Source: CAD feature listing. Evaluate the final solid. Frame: model axes, mm. Face numbers are marked on the shaded views. A direction names the side the tool comes from. Give positions to 0.01 mm unless a question says otherwise; leave off trailing zeros. Order: outer loops, then holes, each group sorted by start corner. A loop starts at its lowest first (then second) coordinate and runs counter-clockwise, first axis right, second up. Notation, with made-up numbers: (78, 11) - (107, 11) arc R21 cw to (107, 43) - close; hole circle Ø1 at (-26.5, 59.5). An arc over 180 degrees is marked (long way). Use CSV: the item, a comma, the result in double quotes.
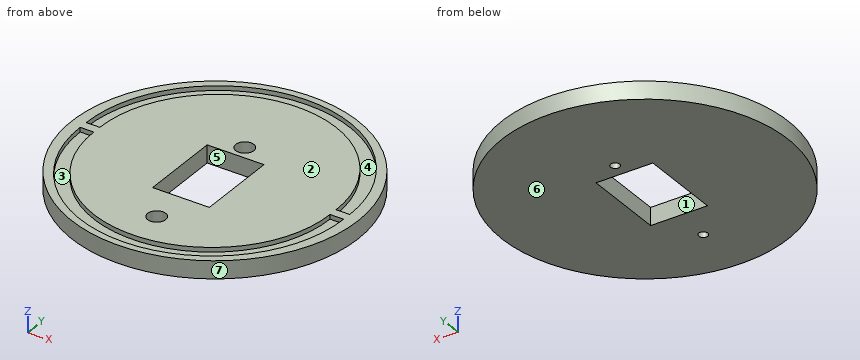
```python
from build123d import *

# Parameters (mm, degrees)
CROQUIS1_R              = 31.5
SALIENTE_EXTRUIR1_DEPTH = 2.4
CROQUIS2_W              = 16.1
CROQUIS2_H              = 36.6
CROQUIS2_W_2            = 12.5
CROQUIS2_H_2            = 33
SALIENTE_EXTRUIR2_DEPTH = 22.5
CROQUIS5_W              = 16.1
CROQUIS5_H              = 36.6
CORTAR_EXTRUIR2_DEPTH   = 9
CROQUIS6_R              = 1.5
CORTAR_EXTRUIR3_DEPTH   = 2.4
CROQUIS7_W              = 12.5
CROQUIS7_H              = 9
SALIENTE_EXTRUIR3_DEPTH = 33
CROQUIS8_R              = 1
CORTAR_EXTRUIR5_DEPTH   = 9
SALIENTE_EXTRUIR4_DEPTH = 12.5
CROQUIS10_W             = 4
CROQUIS10_H             = 2
CORTAR_EXTRUIR6_DEPTH   = 9
CROQUIS11_R             = 31.5
CROQUIS11_W             = 12.5
CROQUIS11_H             = 18
SALIENTE_EXTRUIR5_DEPTH = 3.9
CORTAR_EXTRUIR7_START   = 7
CROQUIS12_R             = 1
CORTAR_EXTRUIR7_DEPTH   = 3.9
CROQUIS13_R             = 2
CORTAR_EXTRUIR8_DEPTH   = 2.4
CROQUIS14_R             = 31.5
CORTAR_EXTRUIR9_DEPTH   = 24.9
CROQUIS15_R             = 31.5
CROQUIS15_R_2           = 2
CROQUIS15_W             = 12.5
CROQUIS15_H             = 18
SALIENTE_EXTRUIR6_DEPTH = 1
CORTAR_EXTRUIR10_DEPTH  = 2
CROQUIS17_R             = 31.5
CORTAR_EXTRUIR11_DEPTH  = 1


with BuildPart() as part:
    # Croquis1 → Saliente-Extruir1 (new body)
    with BuildSketch(Plane.XY):
        with Locations((-51.235671923, 9.786589019)):
            Circle(CROQUIS1_R)
    extrude(amount=SALIENTE_EXTRUIR1_DEPTH)

    # Croquis2 → Saliente-Extruir2 (add)
    with BuildSketch(Plane.XY.offset(2.4)):
        with Locations((-51.235671923, 5.086589019)):
            Rectangle(CROQUIS2_W, CROQUIS2_H)
        with Locations((-51.235671923, 5.086589019)):
            Rectangle(CROQUIS2_W_2, CROQUIS2_H_2, mode=Mode.SUBTRACT)
    extrude(amount=SALIENTE_EXTRUIR2_DEPTH)

    # Croquis5 → Cortar-Extruir2 (cut)
    with BuildSketch(Plane.XY.offset(2.4)):
        with Locations((-51.235671923, 5.086589019)):
            Rectangle(CROQUIS5_W, CROQUIS5_H)
    extrude(amount=-CORTAR_EXTRUIR2_DEPTH, mode=Mode.SUBTRACT)


with BuildPart() as cortar_extruir2_piece_1:
    # of the separate pieces the step leaves, piece 1, a body of its own (cortar_extruir2_pieces)
    add(part.part.solids().sort_by_distance((-19.735671923, 9.786589019, 0))[0])

    # Croquis6 → Cortar-Extruir3 (cut)
    with BuildSketch(Plane(origin=(0, 0, 0), x_dir=(-1, 0, 0), z_dir=(0, 0, -1))):
        with Locations((34.618662565, 26.403598377)):
            Circle(CROQUIS6_R)
        with Locations((67.85268128, 26.403598377)):
            Circle(CROQUIS6_R)
        with Locations((67.85268128, -6.830420339)):
            Circle(CROQUIS6_R)
        with Locations((34.618662565, -6.830420339)):
            Circle(CROQUIS6_R)
        Polygon((51.235671923, 23.386589019), (53.235671923, 23.386589019), (53.235671923, 43.386589019), (49.235671923, 43.386589019), (49.235671923, 23.386589019), align=None)
    extrude(amount=-CORTAR_EXTRUIR3_DEPTH, mode=Mode.SUBTRACT)


with BuildPart() as cortar_extruir2_piece_2:
    # of the separate pieces the step leaves, piece 2, a body of its own (cortar_extruir2_pieces)
    add(part.part.solids().sort_by_distance((-59.285671923, -13.213410981, 24.9))[0])

    # Croquis7 → Saliente-Extruir3 (add)
    with BuildSketch(Plane.XZ.offset(-21.586589019)):
        with Locations((-51.235671923, 13.4)):
            Rectangle(CROQUIS7_W, CROQUIS7_H)
    extrude(amount=SALIENTE_EXTRUIR3_DEPTH)

    # Croquis8 → Cortar-Extruir5 (cut)
    with BuildSketch(Plane.XY.offset(17.9)):
        with Locations((-51.235671923, -9.413410981)):
            Circle(CROQUIS8_R)
        with Locations((-51.235671923, 19.636589019)):
            Circle(CROQUIS8_R)
        Polygon((-44.985671923, -6.413410981), (-57.485671923, -6.413410981), (-57.485671923, 16.586589019), (-53.235671923, 16.586589019), (-53.235671923, 18.586589019), (-49.235671923, 18.586589019), (-49.235671923, 16.586589019), (-44.985671923, 16.586589019), align=None)
    extrude(amount=-CORTAR_EXTRUIR5_DEPTH, mode=Mode.SUBTRACT)

    # Croquis9 → Saliente-Extruir4 (add)
    with BuildSketch(Plane.ZY.offset(44.985671923)):
        Polygon((8.9, -6.413410981), (3.9, -11.413410981), (8.9, -11.413410981), align=None)
        Polygon((8.9, 16.586589019), (3.9, 21.586589019), (8.9, 21.586589019), align=None)
    extrude(amount=SALIENTE_EXTRUIR4_DEPTH)

    # Croquis10 → Cortar-Extruir6 (cut)
    with BuildSketch(Plane.XY.offset(8.9)):
        with Locations((-51.235671923, 17.586589019)):
            Rectangle(CROQUIS10_W, CROQUIS10_H)
    extrude(amount=-CORTAR_EXTRUIR6_DEPTH, mode=Mode.SUBTRACT)

    # Croquis11 → Saliente-Extruir5 (add)
    with BuildSketch(Plane.XY.offset(24.9)):
        with Locations((-51.235671923, 9.786589019)):
            Circle(CROQUIS11_R)
        with Locations((-51.235671923, 7.586589019)):
            Rectangle(CROQUIS11_W, CROQUIS11_H, mode=Mode.SUBTRACT)
    extrude(amount=SALIENTE_EXTRUIR5_DEPTH)

    # Croquis12 → Cortar-Extruir7 (cut)
    with BuildSketch(Plane.XY.offset(17.9).offset(CORTAR_EXTRUIR7_START)):
        with Locations((-51.235671923, 19.636589019)):
            Circle(CROQUIS12_R)
        with Locations((-51.235671923, -9.413410981)):
            Circle(CROQUIS12_R)
    extrude(amount=CORTAR_EXTRUIR7_DEPTH, mode=Mode.SUBTRACT)

    # Croquis13 → Cortar-Extruir8 (cut)
    with BuildSketch(Plane.XY.offset(28.8)):
        with Locations((-51.235671923, 19.636589019)):
            Circle(CROQUIS13_R)
        with Locations((-51.235671923, -9.413410981)):
            Circle(CROQUIS13_R)
    extrude(amount=-CORTAR_EXTRUIR8_DEPTH, mode=Mode.SUBTRACT)


with BuildPart() as cortar_extruir9_tool:
    # Croquis14 → Cortar-Extruir9 (new body)
    with BuildSketch(Plane(origin=(0, 0, 0), x_dir=(-1, 0, 0), z_dir=(0, 0, -1))):
        with Locations(Location((51.235671923, 9.786589019, 0), (0, 0, 180))):
            Circle(CROQUIS14_R)
    extrude(amount=-CORTAR_EXTRUIR9_DEPTH)


with BuildPart() as cortar_extruir2_piece_1_1:
    add(cortar_extruir2_piece_1.part)

    # Cortar-Extruir9: cut by cortar_extruir9_tool
    add(cortar_extruir9_tool.part, mode=Mode.SUBTRACT)


with BuildPart() as cortar_extruir2_piece_2_1:
    add(cortar_extruir2_piece_2.part)

    # Cortar-Extruir9: cut by cortar_extruir9_tool
    add(cortar_extruir9_tool.part, mode=Mode.SUBTRACT)

    # Croquis15 → Saliente-Extruir6 (add)
    with BuildSketch(Plane.XY.offset(28.8)):
        with Locations((-51.235671923, 9.786589019)):
            Circle(CROQUIS15_R)
        with Locations((-51.235671923, 19.636589019)):
            Circle(CROQUIS15_R_2, mode=Mode.SUBTRACT)
        with Locations((-51.235671923, -9.413410981)):
            Circle(CROQUIS15_R_2, mode=Mode.SUBTRACT)
        with Locations((-51.235671923, 7.586589019)):
            Rectangle(CROQUIS15_W, CROQUIS15_H, mode=Mode.SUBTRACT)
    extrude(amount=SALIENTE_EXTRUIR6_DEPTH)

    # Croquis16 → Cortar-Extruir10 (cut)
    with BuildSketch(Plane.XY.offset(29.8)):
        with BuildLine():
            Line((-22.235671923, 8.786589019), (-25.235671923, 8.786589019))
            ThreePointArc((-25.235671923, 8.786589019), (-51.235671923, -17.213410981), (-77.235671923, 8.786589019))
            Line((-77.235671923, 8.786589019), (-80.235671923, 8.786589019))
            ThreePointArc((-80.235671923, 8.786589019), (-51.235671923, -20.213410981), (-22.235671923, 8.786589019))
        make_face()
        with BuildLine():
            Line((-22.235671923, 10.786589019), (-25.235671923, 10.786589019))
            ThreePointArc((-25.235671923, 10.786589019), (-51.235671923, 36.786589019), (-77.235671923, 10.786589019))
            Line((-77.235671923, 10.786589019), (-80.235671923, 10.786589019))
            ThreePointArc((-80.235671923, 10.786589019), (-51.235671923, 39.786589019), (-22.235671923, 10.786589019))
        make_face()
    extrude(amount=-CORTAR_EXTRUIR10_DEPTH, mode=Mode.SUBTRACT)

    # Croquis17 → Cortar-Extruir11 (cut)
    with BuildSketch(Plane.XY.offset(29.8)):
        with Locations((-51.235671923, 9.786589019)):
            Circle(CROQUIS17_R)
    extrude(amount=-CORTAR_EXTRUIR11_DEPTH, mode=Mode.SUBTRACT)


solid = cortar_extruir2_piece_2_1.part
```
Item 1: First-contact query: pin 1 (1.2 mm diameter, centred on x = -51, y = -8.5, fed in from +Z); pin 2 (0.5 mm diameter, centred on x = -78.5, z = 28.5, fed in from -Y). Flat tips, straight axial feed; report the tip coordinate or a pass-through.
Filled in:
pin 1,"stops at z = 26.4"
pin 2,"stops at y = -6.41"
Item 2: Set-up query: the marked faces 1, 2 and 3. Return all of +Z, -Z, +X, -X, +Y, -Y with unobstructed straight access to the full face (end or side cutting, diameter ignored); none if empty.
Filled in:
face 1,"+Z, -Z"
face 2,"+Z, +X, -X, +Y, -Y"
face 3,"+Z"
Item 3: Section D-D on x = -48. Return the cut outline in (y, z), then the cut area to 3 significant figures.
Filled in:
outline,"(-21.55, 24.9) - (-1.41, 24.9) - (-1.41, 28.8) - (-17.01, 28.8) - (-17.01, 27.8) - (-20.03, 27.8) - (-20.03, 28.8) - (-21.55, 28.8) - close; (16.59, 24.9) - (41.12, 24.9) - (41.12, 28.8) - (39.61, 28.8) - (39.61, 27.8) - (36.58, 27.8) - (36.58, 28.8) - (16.59, 28.8) - close"
area,"168 mm2"
Item 4: Section C-C on x = -79. Return the cut outline in (y, z), then the cut area to 3 significant figures.
Filled in:
outline,"(-5.09, 24.9) - (24.67, 24.9) - (24.67, 28.8) - (19.16, 28.8) - (19.16, 27.8) - (10.79, 27.8) - (10.79, 28.8) - (8.79, 28.8) - (8.79, 27.8) - (0.41, 27.8) - (0.41, 28.8) - (-5.09, 28.8) - close"
area,"99.3 mm2"
Item 5: Section B-B on z = 25.5. Return the cut outline in (x, y), then the cut area to 3 significant figures.
Filled in:
outline,"circle Ø63 at (-51.24, 9.79); hole (-57.49, -1.41) - (-44.99, -1.41) - (-44.99, 16.59) - (-57.49, 16.59) - close; hole circle Ø2 at (-51.24, -9.41); hole circle Ø2 at (-51.24, 19.64)"
area,"2,890 mm2"
Item 6: Material intervals for line 1 (Y direction, x = -60, z = 28); line 2 (Y direction, x = -50.5, z = 27.15); line 3 (Y direction, x = -55.5, z = 28.45), sorted ascending. Write a range as from..to.
Filled in:
line 1,"y = -20.47..-18.86, -15.69..35.26, 38.43..40.04"
line 2,"y = -21.7..-11.27, -7.55..-1.41, 16.59..17.78, 21.5..41.28"
line 3,"y = -21.42..-19.9, -16.86..-1.41, 16.59..36.43, 39.47..41"
Item 7: Section A-A on y = 7. Return the cut outline in (x, z), then the cut area to 3 significant figures.
Filled in:
outline,"(-82.61, 24.9) - (-57.49, 24.9) - (-57.49, 28.8) - (-77.17, 28.8) - (-77.17, 27.8) - (-80.18, 27.8) - (-80.18, 28.8) - (-82.61, 28.8) - close; (-44.99, 24.9) - (-19.86, 24.9) - (-19.86, 28.8) - (-22.29, 28.8) - (-22.29, 27.8) - (-25.3, 27.8) - (-25.3, 28.8) - (-44.99, 28.8) - close"
area,"190 mm2"
Item 8: Mould query, pull axis X, two halves, no side actions, for the marked faces 4, 5, 6 and 7. Classes: released by +X, released by -X, zero draft, split by the parting line, or undercut.
Filled in:
face 4,"undercut"
face 5,"undercut"
face 6,"zero draft"
face 7,"split by the parting line"
